```python
from build123d import *

# Parameters (mm, degrees)
SKETCH1_R           = 4.08
BOSS_EXTRUDE1_DEPTH = 8.65
CUT_EXTRUDE1_START  = -1
SKETCH2_R           = 5.08
CUT_EXTRUDE1_DEPTH  = 4.4
FILLET1_R           = 2
FILLET2_R           = 1


with BuildPart() as part:
    # Sketch1 → Boss-Extrude1 (new body)
    with BuildSketch(Plane(origin=(0, 0, 0), x_dir=(1, 0, 0), z_dir=(0, 1, 0))):
        with BuildLine():
            Line((-20, 7), (20, 7))
            ThreePointArc((20, 7), (27, 0), (20, -7))
            Line((20, -7), (-20, -7))
            ThreePointArc((-20, -7), (-27, 0), (-20, 7))
        make_face()
        with Locations((-20, 0)):
            Circle(SKETCH1_R, mode=Mode.SUBTRACT)
        with Locations((20, 0)):
            Circle(SKETCH1_R, mode=Mode.SUBTRACT)
    extrude(amount=BOSS_EXTRUDE1_DEPTH)

    # Sketch2 → Cut-Extrude1 (cut)
    with BuildSketch(Plane.XZ.offset(CUT_EXTRUDE1_START)):
        with Locations((-20, 0)):
            Circle(SKETCH2_R)
        with Locations((20, 0)):
            Circle(SKETCH2_R)
    extrude(amount=-CUT_EXTRUDE1_DEPTH, mode=Mode.SUBTRACT)

    # Fillet1
    fillet1_edges = [part.edges().sort_by_distance(p)[0] for p in [
        (27, 8.65, 0),
        (0, 8.65, -7),
        (-27, 8.65, 0),
        (0, 0, -7),
        (27, 0, 0),
        (0, 0, 7),
        (-27, 0, 0),
        (0, 8.65, 7),
    ]]
    fillet(fillet1_edges, radius=FILLET1_R)

    # Fillet2
    fillet2_edges = [part.edges().sort_by_distance(p)[0] for p in [
        (-24.08, 8.65, 0),
        (15.92, 8.65, 0),
    ]]
    fillet(fillet2_edges, radius=FILLET2_R)


solid = part.part
```
Geometry check sheet. Reference: the model listing, model coordinates, mm. A direction names the side the tool comes from. Coordinates: 2 decimals unless noted, no trailing zeros. Order: outer loops, then holes, each group sorted by start corner. A loop starts at its lowest first (then second) coordinate and runs counter-clockwise, first axis right, second up. Notation, with made-up numbers: (-28.75, 53.25) - (2.25, 53.25) arc R10 ccw to (2.25, 61.25) - close; hole circle Ø3 at (-16.5, -31.5). An arc over 180 degrees is marked (long way). Answer as a JSON object with one key per item and string values. Group by question number.
Item 1: Depth check by flat-ended pin: pin 1 Ø5 at (y, z) = (4.5, 4) entering from +X. Enter the tip coordinate at first touch or a pass-through.
Item 2: Sectioned sample at B-B, the plane x = -3. Record the cut outline in (y, z), and give its area (3 significant figures).
Item 3: Tool access check on faces 4 (the face through (20.7, 1, 4.2)), 5 (the face through (-0.28, 8.05, 6.43)). Record the directions out of +Z, -Z, +X, -X, +Y, -Y that give a thin tool (end or side, any length) a straight path to the whole face; none if there is none.
Item 4: Sectioned sample at C-C, the plane z = 3. Give the number of separate pieces and of enclosed holes in the cut face, and give its area (3 significant figures).
Item 5: Draft check along Y on faces 1 (the face through (0.28, 0.6, -6.43)), 2 (the face through (23.77, 0.49, 1.56)), 3 (the face through (20.7, 5.4, 4.2)). Enter one of: +Y half, -Y half, draft (parallel to the pull), parting line (faces both ways), or undercut.
Item 6: Scan lines: probe 1 along X at (y, z) = (6.5, 0); probe 2 along Z at (x, y) = (20, 2.05); probe 3 along Z at (x, y) = (-20, 6.5). Record each from-to range of solid material in increasing order.
Item 7: Sectioned sample at A-A, the plane y = 4.25. Record the cut outline in (x, z).
Resolved:
{
 "1": {"pin 1": "x = 26.84"},
 "2": {"outline": "(0, -5) arc R2 ccw to (2, -7) - (6.65, -7) arc R2 ccw to (8.65, -5) - (8.65, 5) arc R2 ccw to (6.65, 7) - (2, 7) arc R2 ccw to (0, 5) - close", "area": "118 mm^2"},
 "3": {"face 4": "none", "face 5": "+Z, +X, -X, +Y"},
 "4": {"separate pieces": "3", "enclosed holes": "0", "area": "331 mm^2"},
 "5": {"face 1": "-Y half", "face 2": "draft", "face 3": "undercut"},
 "6": {"probe 1": "-27 to -24.08, -15.92 to 15.92, 24.08 to 27", "probe 2": "-7 to -5.08, 5.08 to 7", "probe 3": "-7 to -4.08, 4.08 to 7"},
 "7": {"outline": "(-20, -7) - (20, -7) arc R7 ccw to (20, 7) - (-20, 7) arc R7 ccw to start; hole circle Ø10.16 at (-20, 0); hole circle Ø10.16 at (20, 0)"}
}
